Read the model definition and answer for the solid it produces. Units are mm, in the model's axes. A direction names the side the tool comes from. Coordinates: 2 decimals unless noted, no trailing zeros. Write each loop counter-clockwise with the first axis right and the second up, starting at its lowest first coordinate (ties: lowest second). Pieces come first, ordered by that corner, then holes. Notation, with made-up numbers: M -6,-3 L 14,-3 A24 cw 14,35 Z; hole C 38,-13 d5. An arc over 180 degrees is marked long. Write item = value, one per line.
from build123d import *


with BuildPart() as f1:
    # F0 (on Front) → F1 (revolve)
    with BuildSketch(Plane.XZ):
        with BuildLine():
            Line((-7.9375, 0), (-3.175, 0))
            Line((-3.175, 0), (-3.175, 3.175))
            Line((-3.175, 3.175), (-7.2748389157, 3.175))
            ThreePointArc((-7.2748389157, 3.175), (-7.7700688589, 1.6217077968), (-7.9375, 0))
        make_face()
        with BuildLine():
            Line((-3.175, -3.175), (-3.175, 0))
            Line((-3.175, 0), (-7.9375, 0))
            ThreePointArc((-7.9375, 0), (-7.7700688589, -1.6217077968), (-7.2748389157, -3.175))
            Line((-7.2748389157, -3.175), (-3.175, -3.175))
        make_face()
        with BuildLine():
            Line((-3.175, 3.175), (-3.175, 7.2748389157))
            ThreePointArc((-3.175, 7.2748389157), (-5.6126600757, 5.6126600757), (-7.2748389157, 3.175))
            Line((-7.2748389157, 3.175), (-3.175, 3.175))
        make_face()
        with BuildLine():
            ThreePointArc((-7.2748389157, -3.175), (-5.6126600757, -5.6126600757), (-3.175, -7.2748389157))
            Line((-3.175, -7.2748389157), (-3.175, -3.175))
            Line((-3.175, -3.175), (-7.2748389157, -3.175))
        make_face()
    revolve(axis=Axis((0, 0, -5.1538590342), (0, 0, -1)))

    # F0 (on Front) → F2 (revolve)
    with BuildSketch(Plane.XZ):
        with BuildLine():
            Line((-20.6375, 0), (-7.9375, 0))
            ThreePointArc((-7.9375, 0), (-7.7700688589, 1.6217077968), (-7.2748389157, 3.175))
            Line((-7.2748389157, 3.175), (-21.8502420857, 3.175))
            ThreePointArc((-21.8502420857, 3.175), (-20.9510041404, 1.6993652025), (-20.6375, 0))
        make_face()
        with BuildLine():
            ThreePointArc((7.2748389157, 3.175), (7.7700688589, 1.6217077968), (7.9375, 0))
            Line((7.9375, 0), (20.6375, 0))
            ThreePointArc((20.6375, 0), (20.9510041404, 1.6993652025), (21.8502420857, 3.175))
            Line((21.8502420857, 3.175), (7.2748389157, 3.175))
        make_face()
        with BuildLine():
            Line((-30.1625, 0), (-25.4, 0))
            Line((-25.4, 0), (-25.4, 3.175))
            Line((-25.4, 3.175), (-25.4, 4.7625))
            ThreePointArc((-25.4, 4.7625), (-26.36557418, 4.6635901142), (-27.2910413441, 4.3709688726))
            ThreePointArc((-27.2910413441, 4.3709688726), (-29.3804202448, 2.6148921439), (-30.1625, 0))
        make_face()
        with BuildLine():
            Line((-25.4, 0), (-20.6375, 0))
            ThreePointArc((-20.6375, 0), (-20.9510041404, 1.6993652025), (-21.8502420857, 3.175))
            Line((-21.8502420857, 3.175), (-25.4, 3.175))
            Line((-25.4, 3.175), (-25.4, 0))
        make_face()
        with BuildLine():
            Line((-25.4, 3.175), (-21.8502420857, 3.175))
            ThreePointArc((-21.8502420857, 3.175), (-23.4557175167, 4.3475478002), (-25.4, 4.7625))
            Line((-25.4, 4.7625), (-25.4, 3.175))
        make_face()
        with BuildLine():
            ThreePointArc((21.8502420857, 3.175), (20.9510041404, 1.6993652025), (20.6375, 0))
            Line((20.6375, 0), (25.4, 0))
            Line((25.4, 0), (25.4, 3.175))
            Line((25.4, 3.175), (21.8502420857, 3.175))
        make_face()
        with BuildLine():
            ThreePointArc((25.4, 4.7625), (23.4557175167, 4.3475478002), (21.8502420857, 3.175))
            Line((21.8502420857, 3.175), (25.4, 3.175))
            Line((25.4, 3.175), (25.4, 4.7625))
        make_face()
        with BuildLine():
            Line((25.4, 3.175), (25.4, 0))
            Line((25.4, 0), (30.1625, 0))
            ThreePointArc((30.1625, 0), (29.3804202448, 2.6148921439), (27.2910413441, 4.3709688726))
            ThreePointArc((27.2910413441, 4.3709688726), (26.36557418, 4.6635901142), (25.4, 4.7625))
            Line((25.4, 4.7625), (25.4, 3.175))
        make_face()
    revolve(axis=Axis((0.3062523901, 0, 0), (1, 0, 0)))

    # F0 (on Front) → F3 (revolve)
    with BuildSketch(Plane.XZ):
        with BuildLine():
            ThreePointArc((-27.2910413441, 4.3709688726), (-26.36557418, 4.6635901142), (-25.4, 4.7625))
            Line((-25.4, 4.7625), (-25.4, 36.5125))
            add(Edge.make_bspline(
                [(-25.4, 36.5125), (-26.816893369, 36.1733324826), (-29.9766271953, 30.3995680819), (-30.0177491556, 22.0177094067), (-26.5618020908, 13.4239134261), (-28.2605474591, 5.8526801132), (-27.5281520721, 4.7952938673), (-27.2910413441, 4.3709688726)],
                knots=[0, 0, 0, 0, 0.2074904054, 0.4438338536, 0.6895354369, 0.9020581403, 1, 1, 1, 1], degree=3))
        make_face()
    revolve(axis=Axis((-25.4, 0, 14.7146796808), (0, 0, -1)))

    # F0 (on Front) → F4 (revolve)
    with BuildSketch(Plane.XZ):
        with BuildLine():
            Line((25.4, 36.5125), (25.4, 4.7625))
            ThreePointArc((25.4, 4.7625), (26.36557418, 4.6635901142), (27.2910413441, 4.3709688726))
            add(Edge.make_bspline(
                [(25.4, 36.5125), (26.816893369, 36.1733324826), (29.9766271953, 30.3995680819), (30.0177491556, 22.0177094067), (26.5618020908, 13.4239134261), (28.2605474591, 5.8526801132), (27.5281520721, 4.7952938673), (27.2910413441, 4.3709688726)],
                knots=[0, 0, 0, 0, 0.2074904054, 0.4438338536, 0.6895354369, 0.9020581403, 1, 1, 1, 1], degree=3))
        make_face()
    revolve(axis=Axis((25.4, 0, 13.9341913164), (0, 0, -1)))


solid = f1.part
Item 1: Flat-ended cylindrical pins translate along their axes: pin 1 (1.5 mm diameter, centred on y = 4.5, z = 26.5, fed in from +X); pin 2 (5 mm diameter, centred on x = 21, z = 22, fed in from +Y); pin 3 (7.5 mm diameter, centred on x = 0, y = 0, fed in from +Z). Find the tip coordinate at first contact, or state that the pin passes through.
Worked answers:
pin_1 = 27.72
pin_2 = 3.63
pin_3 = 7.27
Item 2: Find section B-B (x = 11.5). Determine the outline of the cut face in (y, z) (3 decimals), and give its area (3 significant figures).
Worked answers:
outline = C 0,0 d6.35
area = 31.7 mm²
Item 3: Which of the six approach directions +Z, -Z, +X, -X, +Y, -Y give full straight-line access (tool end or side, diameter ignored) to faces 1 (the face through (14.46, 3.1, -0.69)), 2 (the face through (0.69, -3.1, 0.1))?
Worked answers:
face_1 = none
face_2 = +Z, -Z
Item 4: Find section A-A (x = 0). Determine the outline of the cut face in (y, z) (1 decimal).
Worked answers:
outline = M -3.2,-7.3 L -3.2,7.3 A7.9 ccw Z; M 3.2,-7.3 A7.9 ccw 3.2,7.3 Z
Item 5: Find section C-C (y = 6.5). Determine the outline of the cut face in (x, z) (3 decimals), and give its area (3 significant figures).
Worked answers:
outline = C 0,0 d9.111
area = 65.2 mm²
Item 6: Consider line 1 along X through (y, z) = (-2, 21.5); line 2 along Y through (x, z) = (0, -0.25) (3 decimals); line 3 along Y through (x, z) = (0, -3.25) (3 decimals). Determine where each line is inside the solid, lowest interval first. Write a range as from..to.
Worked answers:
line_1 = -28.76..-22.04, 22.04..28.76
line_2 = -7.934..-3.175, 3.175..7.934
line_3 = -7.242..-3.175, 3.175..7.242
